from build123d import *

# Parameters (mm, degrees)
F0_W     = 5.25
F0_H     = 50.25
F0_W_2   = 137.75
F0_H_2   = 20.25
F0_W_3   = 50.5
F0_H_3   = 5.25
F0_H_4   = 4.25
F0_W_4   = 20.5
F0_H_5   = 20.5
F0_W_5   = 4.25
F0_H_6   = 173.25
F0_W_6   = 40.5
F0_H_7   = 40.25
F0_R     = 20
F1_DEPTH = 1
F2_W     = 3
F2_H     = 1
F2_W_2   = 93.75
F2_W_3   = 6
F2_H_2   = 6
F3_DEPTH = 25


with BuildPart() as f1:
    # F0 (on Top) → F1 (new body)
    with BuildSketch(Plane.XY):
        with Locations((-231.875, -87.375)):
            Rectangle(F0_W, F0_H)
        with Locations((-68.875, -122.625)):
            Rectangle(F0_W_2, F0_H_2)
        with Locations((-183.5, -39.125)):
            Rectangle(F0_W_3, F0_H_3)
        with Locations((-68.875, 113.125)):
            Rectangle(F0_W_2, F0_H_4)
        with Locations((-219, -87.375)):
            Rectangle(F0_W_4, F0_H)
        with Locations((-183.5, -52)):
            Rectangle(F0_W_3, F0_H_5)
        with Locations((-139.875, 24.375)):
            Rectangle(F0_W_5, F0_H_6)
        Polygon((-137.75, -112.5), (-137.75, -62.25), (-142, -62.25), (-158.25, -62.25), (-158.25, -112.5), align=None)
        with Locations((-183.5, -87.375)):
            Rectangle(F0_W_3, F0_H)
        with Locations((-183.5, -87.375)):
            Rectangle(F0_W_6, F0_H_7, mode=Mode.SUBTRACT)
        Polygon((0, 102), (0, 111), (-137.75, 111), (-137.75, -62.25), (-137.75, -112.5), (0, -112.5), (0, -45), (-128.75, -45), (-128.75, 102), align=None)
        with Locations((-112.75, -87.5)):
            Circle(F0_R, mode=Mode.SUBTRACT)
    extrude(amount=F1_DEPTH)

    # F2 (on face) → F3 (cut)
    with BuildSketch(Plane.XY.offset(1)):
        Polygon((-134.75, -115.5), (-134.75, -109.5), (-140.75, -109.5), (-140.75, -111.5), (-137.75, -111.5), (-137.75, -112.5), (-140.75, -112.5), (-140.75, -115.5), align=None)
        with Locations((-139.25, -112)):
            Rectangle(F2_W, F2_H)
        with Locations((-187.625, -112)):
            Rectangle(F2_W_2, F2_H)
        with Locations((-158.25, -62.25)):
            Rectangle(F2_W_3, F2_H_2)
        with Locations((-208.75, -62.25)):
            Rectangle(F2_W_3, F2_H_2)
        with Locations((-137.75, 111)):
            Rectangle(F2_W_3, F2_H_2)
    extrude(amount=-F3_DEPTH, mode=Mode.SUBTRACT)


solid = f1.part
Can you work these out from the model? Positions are in its coordinate system, mm. Give positions to 0.01 mm unless a question says otherwise; leave off trailing zeros. Loops run counter-clockwise (first coordinate to the right, second up) from the corner with the lowest first, then second, coordinate; pieces in that order, holes last. Notation, with made-up numbers: (78, -33) - (116, -33) arc R23 ccw to (116, -3) - close; hole circle Ø7 at (-36, 89.25). An arc over 180 degrees is marked (long way). Return JSON: item names as keys, results as strings.
1. If I drill on line 1 (Y direction, x = -112.75, z = 0.6); line 2 (Y direction, x = -169.5, z = 0.45); line 3 (Y direction, x = -47, z = 0.2), over which ranges is the centre line in solid material (lowest first)?
Output values:
{"line 1": "y = -132.75 to -107.5, -67.5 to -45, 102 to 115.25", "line 2": "y = -111.5 to -107.5, -67.25 to -36.5", "line 3": "y = -132.75 to -45, 102 to 115.25"}
2. I want a section at D-D on y = 28. Please give me the cut outline in (x, z), and give its area (4 significant figures).
Output values:
{"outline": "(-142, 0) - (-128.75, 0) - (-128.75, 1) - (-142, 1) - close", "area": "13.25 mm²"}
3. I want a section at C-C on z = 0.25. Give the number of separate pieces and of enclosed holes in the cut face, and give its area (3 significant figures).
Output values:
{"separate pieces": "1", "enclosed holes": "2", "area": "19,000 mm²"}
4. We'd pull the mould along X, two halves only. Please class faces 1 (the face through (-109, -54, 0)), 2 (the face through (-128.6, -99.7, 0.5)): +X half, -X half, draft (parallel to the pull), parting line (faces both ways), or undercut.
Output values:
{"face 1": "draft", "face 2": "undercut"}
5. I'm going to push flat-ended pins straight in: pin 1 Ø0.5 at (y, z) = (-48.5, 0.5) entering from -X; pin 2 Ø0.5 at (x, z) = (-185, 0.5) entering from -Y. Where does each tip first touch, or does it pass through?
Output values:
{"pin 1": "stops at x = -208.75", "pin 2": "stops at y = -111.5"}
6. I want a section at A-A on x = -112.75. Please give me the cut outline in (y, z).
Output values:
{"outline": "(-132.75, 0) - (-107.5, 0) - (-107.5, 1) - (-132.75, 1) - close; (-67.5, 0) - (-45, 0) - (-45, 1) - (-67.5, 1) - close; (102, 0) - (115.25, 0) - (115.25, 1) - (102, 1) - close"}
7. I want a section at B-B on y = -87.5. Please give me the cut outline in (x, z), and give its area (3 significant figures).
Output values:
{"outline": "(-234.5, 0) - (-203.75, 0) - (-203.75, 1) - (-234.5, 1) - close; (-163.25, 0) - (-132.75, 0) - (-132.75, 1) - (-163.25, 1) - close; (-92.75, 0) - (0, 0) - (0, 1) - (-92.75, 1) - close", "area": "154 mm²"}
